Here's the drawing with two shaded views (mm, measured from the low corner). I have some questions. Give positions to 0.01 mm unless a question says otherwise; leave off trailing zeros. Loops run counter-clockwise (first coordinate to the right, second up) from the corner with the lowest first, then second, coordinate; pieces in that order, holes last. Notation, with made-up numbers: M -34,13.25 L -25,13.25 A17 ccw -25,26.25 Z; hole C -37.5,14.5 d1. An arc over 180 degrees is marked long. Answer in a Markdown table with one row per item. Add a question column.
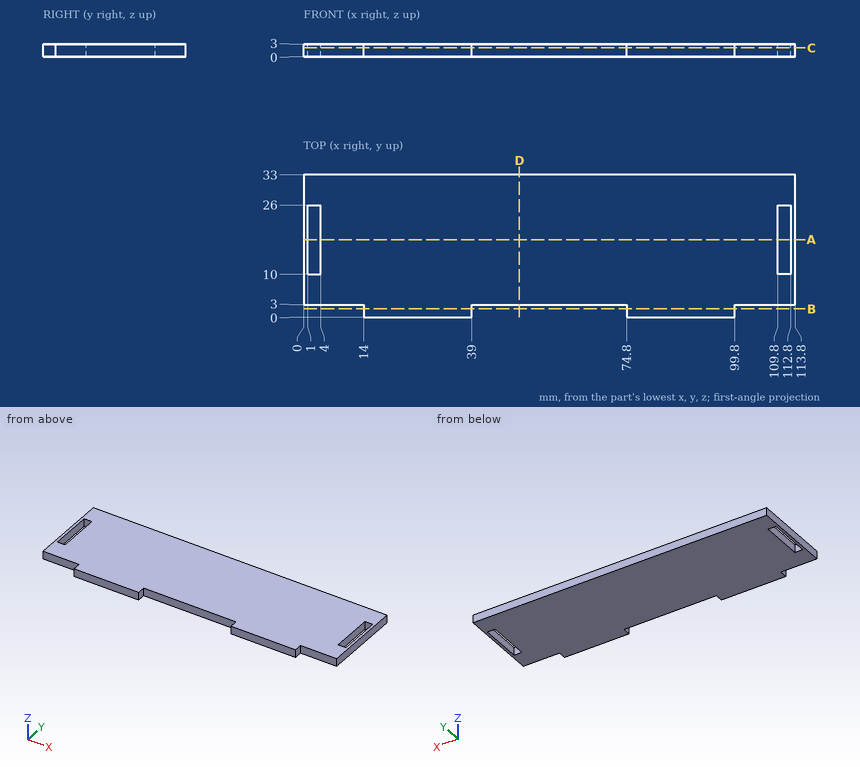
Item 1: Suppose I cut it at D-D (x = 50). List the corners of the cut face in (y, z) for me, then the cut area to 3 significant figures.
Item 2: Suppose I cut it at C-C (z = 2.1). List the corners of the cut face in (x, y) for me, then the cut area to 3 significant figures.
Item 3: I need wall thicknesses on L1, parallel to X at y = 25, z = 0.2; L2, parallel to Y at x = 6, z = 1.2. Which ranges of each line are inside material? Lowest first, please.
Item 4: Suppose I cut it at A-A (y = 18). List the corners of the cut face in (x, z) for me, then the cut area to 3 significant figures.
Item 5: For P1, Ø1.5, axis at y = 2, z = 2, coming from the +X side; P2, Ø0.9, axis at y = 2, z = 1.5, coming from the -X side; P3, Ø0.9, axis at x = 104, z = 1.5, coming from the -Y side, each with a flat end and sliding along its axis, tell me the tip position at first contact or that it passes through.
Item 6: Suppose I cut it at B-B (y = 2). List the corners of the cut face in (x, z) for me.
Values found:
| question | item | result |
|---|---|---|
| 1 | outline | M 3,0 L 33,0 L 33,3 L 3,3 Z |
| 1 | area | 90.0 mm² |
| 2 | outline | M 0,3 L 14,3 L 14,0 L 39,0 L 39,3 L 74.8,3 L 74.8,0 L 99.8,0 L 99.8,3 L 113.8,3 L 113.8,33 L 0,33 Z; hole M 1,10 L 4,10 L 4,26 L 1,26 Z; hole M 109.8,10 L 112.8,10 L 112.8,26 L 109.8,26 Z |
| 2 | area | 3,470 mm² |
| 3 | L1 | 0 to 1, 4 to 109.8, 112.8 to 113.8 |
| 3 | L2 | 3 to 33 |
| 4 | outline | M 0,0 L 1,0 L 1,3 L 0,3 Z; M 4,0 L 109.8,0 L 109.8,3 L 4,3 Z; M 112.8,0 L 113.8,0 L 113.8,3 L 112.8,3 Z |
| 4 | area | 323 mm² |
| 5 | P1 | x = 99.8 |
| 5 | P2 | x = 14 |
| 5 | P3 | y = 3 |
| 6 | outline | M 14,0 L 39,0 L 39,3 L 14,3 Z; M 74.8,0 L 99.8,0 L 99.8,3 L 74.8,3 Z |
